Geometry: final body of the model. Coordinates: model frame, mm. A direction names the side the tool comes from. Give positions to 0.01 mm unless a question says otherwise; leave off trailing zeros. Write each loop counter-clockwise with the first axis right and the second up, starting at its lowest first coordinate (ties: lowest second). Pieces come first, ordered by that corner, then holes. Notation, with made-up numbers: (13, 47) - (31, 47) arc R29 cw to (31, 72) - close; hole circle Ø3 at (60, 73). An arc over 180 degrees is marked (long way). Return JSON: item names as keys, results as strings.
from build123d import *

# Parameters (mm, degrees)
BOSS_EXTRUDE1_DEPTH = 7.5
BOSS_EXTRUDE2_DEPTH = 385
BOSS_EXTRUDE3_DEPTH = 7.5


with BuildPart() as part:
    # Sketch1 → Boss-Extrude1 (new body)
    with BuildSketch(Plane.XY):
        Polygon((0, -2.5), (8.964466094, -2.5), (15.303300859, -8.838834765), (18.838834765, -5.303300859), (11.035533906, 2.5), (0, 2.5), align=None)
    extrude(amount=BOSS_EXTRUDE1_DEPTH)

    # Sketch2 → Boss-Extrude2 (add)
    with BuildSketch(Plane.XY.offset(7.5)):
        Polygon((15.126524164, -9.01561146), (20.783378413, -14.67246571), (17.424621202, -18.03122292), (6.893398282, -7.5), (-8, -7.5), (-8, -2.875), (0, -2.875), (0, 2.875), (-8, 2.875), (-8, 7.5), (13.106601718, 7.5), (28.03122292, -7.424621202), (24.67246571, -10.783378413), (19.01561146, -5.126524164), align=None)
    extrude(amount=BOSS_EXTRUDE2_DEPTH)

    # Sketch4 → Boss-Extrude3 (add)
    with BuildSketch(Plane.XY.offset(392.5)):
        Polygon((15.303300859, -8.838834765), (18.838834765, -5.303300859), (11.035533906, 2.5), (0, 2.5), (0, -2.5), (8.964466094, -2.5), align=None)
    extrude(amount=BOSS_EXTRUDE3_DEPTH)


solid = part.part
Q1. Section query A-A, the plane z = 306.5. Return the cut outline in (x, y) (3 decimals).
Answer key:
{"outline": "(-8, -7.5) - (6.893, -7.5) - (17.425, -18.031) - (20.783, -14.672) - (15.127, -9.016) - (19.016, -5.127) - (24.672, -10.783) - (28.031, -7.425) - (13.107, 7.5) - (-8, 7.5) - (-8, 2.875) - (0, 2.875) - (0, -2.875) - (-8, -2.875) - close"}
Q2. Set-up query: faces 1 (the flat face through (11, 3, 7.5)), 2 (the flat face through (4, -2.5, 4)), 3 (the flat face through (4, -2.5, 396)). Return all of +Z, -Z, +X, -X, +Y, -Y with unobstructed straight access to the full face (end or side cutting, diameter ignored); none if empty.
Answer key:
{"face 1": "-Z, +X, +Y", "face 2": "-Z, -X, -Y", "face 3": "+Z, -X, -Y"}
Q3. Mould query, pull axis Y, two halves, no side actions, for faces 4 (the flat face through (9, -2, 400)), 5 (the flat face through (14.992, -1.456, 3.698)), 6 (the flat face through (-4, 2.875, 197)). Classes: pulls with the +Y half, pulls with the -Y half, needs draft (parallel to the pull), parting line crosses it, or undercut.
Answer key:
{"face 4": "needs draft", "face 5": "pulls with the +Y half", "face 6": "undercut"}
Q4. Pin query (flat end, axial travel): P1, Ø7.5, axis at x = 0, z = 198, coming from the -Y side; P2, Ø6, axis at x = 5.5, z = 2.5, coming from the +Y side; P3, Ø12, axis at x = -3, y = -4, coming from the -Z side; P4, Ø1.5, axis at x = 16, y = -14.5, coming from the +Z side. Return the tip coordinate at first contact, or that it passes through.
Answer key:
{"P1": "stops at y = -7.5", "P2": "stops at y = 2.5", "P3": "stops at z = 0", "P4": "stops at z = 392.5"}
Q5. Material intervals for probe 1 along Y at (x, z) = (-1.5, 65) (3 decimals); probe 2 along X at (y, z) = (-4, 222.5); probe 3 along Z at (x, y) = (4, -6.5), sorted ascending. Write a range as [from, to].
Answer key:
{"probe 1": "y = [-7.5, -2.875], [2.875, 7.5]", "probe 2": "x = [-8, 24.61]", "probe 3": "z = [7.5, 392.5]"}
